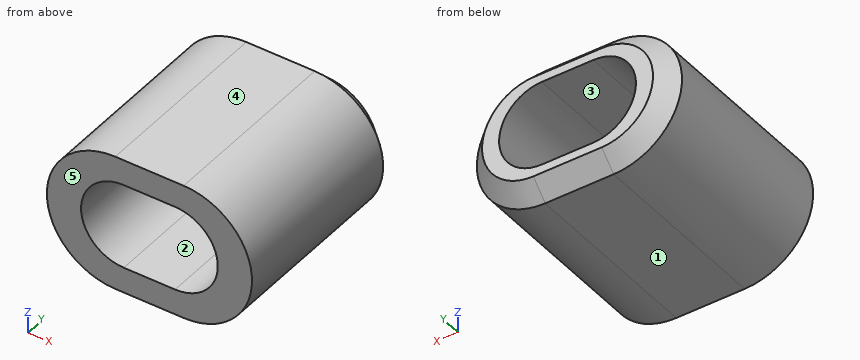
```python
from build123d import *

# Parameters (mm, degrees)
SALIENTE_EXTRUIR1_DEPTH = 60
CHAFL_N1_SIZE           = 5


with BuildPart() as part:
    # Croquis1 → Saliente-Extruir1 (new body)
    with BuildSketch(Plane(origin=(0, 0, 0), x_dir=(1, 0, 0), z_dir=(0, 1, 0))):
        with BuildLine():
            Line((0, -20), (-20, -20))
            ThreePointArc((-20, -20), (-40, 0), (-20, 20))
            Line((-20, 20), (0, 20))
            ThreePointArc((0, 20), (20, 0), (0, -20))
        make_face()
        with BuildLine():
            Line((-2.5, -12.5), (-17.5, -12.5))
            ThreePointArc((-17.5, -12.5), (-30, 0), (-17.5, 12.5))
            Line((-17.5, 12.5), (-2.5, 12.5))
            ThreePointArc((-2.5, 12.5), (10, 0), (-2.5, -12.5))
        make_face(mode=Mode.SUBTRACT)
    extrude(amount=SALIENTE_EXTRUIR1_DEPTH)

    # Chaflán1
    chafl_n1_edges = [part.edges().sort_by_distance(p)[0] for p in [
        (-40, 60, 0),
        (-10, 60, 20),
        (20, 60, 0),
        (-10, 60, -20),
    ]]
    chamfer(chafl_n1_edges, length=CHAFL_N1_SIZE)


solid = part.part
```
Check sheet for the modelled part. Datum: model origin and axes. Units: mm. Face numbers are marked on the shaded views. A direction names the side the tool comes from. Coordinates: 2 decimals unless noted, no trailing zeros. Loops run counter-clockwise (first coordinate to the right, second up) from the corner with the lowest first, then second, coordinate; pieces in that order, holes last. Notation, with made-up numbers: M -37,50.25 L -23,50.25 A24 ccw -23,84.25 Z; hole C -26.5,67.25 d11. An arc over 180 degrees is marked long. Answer as a JSON object with one key per item and string values.
1. Scan lines: L1, parallel to Z at x = -4.5, y = 5; L2, parallel to X at y = 34, z = 10.5; L3, parallel to X at y = 4.5, z = -7.5. Record each from-to range of solid material in increasing order. Write a range as from..to.
Outcome:
{"L1": "-20..-12.5, 12.5..20", "L2": "-37.02..-24.28, 4.28..17.02", "L3": "-38.54..-27.5, 7.5..18.54"}
2. Sectioned sample at A-A on z = 0. Record the cut outline in (x, y).
Outcome:
{"outline": "M -40,0 L -30,0 L -30,60 L -35,60 L -40,55 Z; M 10,0 L 20,0 L 20,55 L 15,60 L 10,60 Z"}
3. Access from +Z, -Z, +X, -X, +Y, -Y to the whole of each face (thin tool, end or side, straight path). Record for the marked faces 1 and 2.
Outcome:
{"face 1": "-Z, +X, -X, +Y, -Y", "face 2": "+Y, -Y"}
4. Depth check by flat-ended pin: P1, Ø4, axis at y = 12, z = 9, coming from the +X side (3 decimals); P2, Ø1.5, axis at y = 22, z = -2, coming from the +X side; P3, Ø12, axis at y = 32.5, z = 9.5, coming from the -X side. Enter the tip coordinate at first touch or a pass-through.
Outcome:
{"P1": "x = 18.735", "P2": "x = 19.96", "P3": "x = -39.69"}
5. Sectioned sample at B-B on y = 15. Record the cut outline in (x, z).
Outcome:
{"outline": "M -20,-20 L 0,-20 A20 ccw 0,20 L -20,20 A20 ccw Z; hole M -17.5,-12.5 L -2.5,-12.5 A12.5 ccw -2.5,12.5 L -17.5,12.5 A12.5 ccw Z"}
6. Release check for a two-part mould opening along Z. For the marked faces 3, 4 and 5 record: pulls with the +Z half, pulls with the -Z half, needs draft (parallel to the pull), parting line crosses it, or undercut.
Outcome:
{"face 3": "undercut", "face 4": "pulls with the +Z half", "face 5": "needs draft"}
